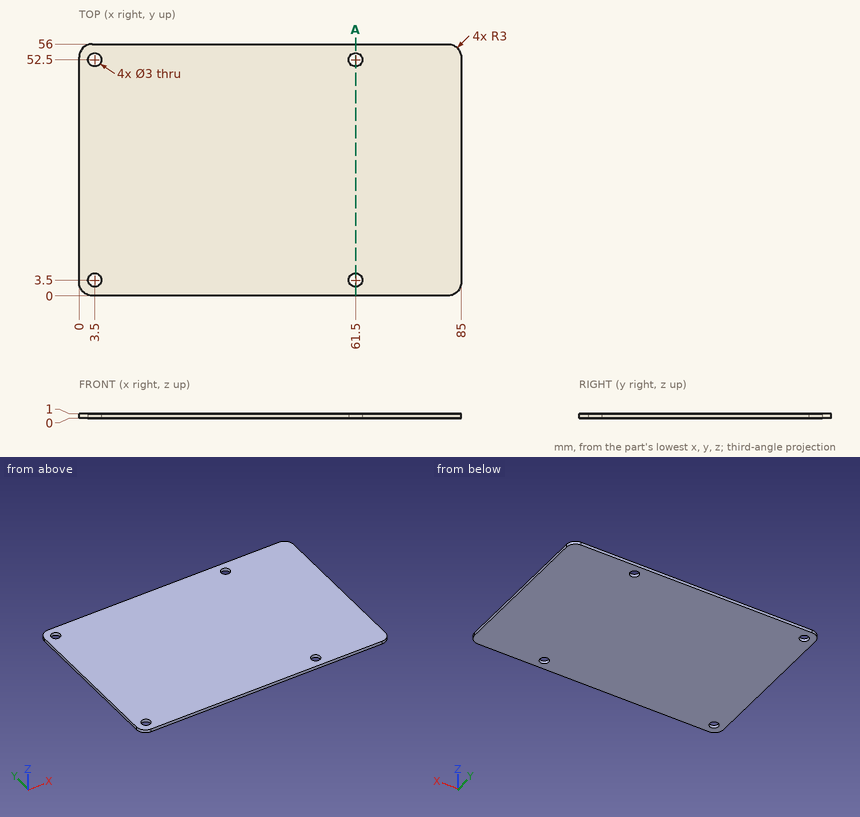
Geometry check sheet. Reference: drawing and pictorial views, mm from the part's lowest x, y, z. Give positions to 0.01 mm unless a question says otherwise; leave off trailing zeros. Order: outer loops, then holes, each group sorted by start corner. A loop starts at its lowest first (then second) coordinate and runs counter-clockwise, first axis right, second up. Notation, with made-up numbers: M 86.5,-5 L 99.5,-5 A24 cw 99.5,11 Z; hole C 89,77.5 d9. An arc over 180 degrees is marked long. Answer as a JSON object with one key per item and string values. Group by question number.
1) Depth check by flat-ended pin: pin 1 Ø1.8 at (x, y) = (61.5, 52.5) entering from -Z. Enter the tip coordinate at first touch or a pass-through.
2) Cross-section at A-A (x = 61.5). Enter the section's corners in (y, z), then the cut area to 3 significant figures.
3) Scan lines: line 1 along X through (y, z) = (52.5, 0.55); line 2 along Y through (x, z) = (61.5, 0.4). Record each from-to range of solid material in increasing order. Write a range as [from, to].
Result sheet:
{
 "1": {"pin 1": "passes through"},
 "2": {"outline": "M 0,0 L 2,0 L 2,1 L 0,1 Z; M 5,0 L 51,0 L 51,1 L 5,1 Z; M 54,0 L 56,0 L 56,1 L 54,1 Z", "area": "50.0 mm2"},
 "3": {"line 1": "x = [0, 2], [5, 60], [63, 85]", "line 2": "y = [0, 2], [5, 51], [54, 56]"}
}
